```python
from build123d import *

# Parameters (mm, degrees)
SKETCH1_W             = 25.4
SKETCH1_H             = 10.668
BOSS_EXTRUDE1_DEPTH   = 5.334
BOSS_EXTRUDE1_2_DEPTH = 5.334
SKETCH1_3_W           = 329.617035208
SKETCH1_3_H           = 10.668
BOSS_EXTRUDE2_DEPTH   = 12.7
DIHEDRAL_ANGLE_DEPTH  = 5.334
SKETCH3_W             = 50.8
SKETCH3_H             = 12.7
CUT_EXTRUDE1_DEPTH    = 5.334


with BuildPart() as part:
    # Sketch1 → Boss-Extrude1 (new body)
    with BuildSketch(Plane(origin=(0, 5.334, 0), x_dir=(1, 0, 0), z_dir=(0, 1, 0))):
        with Locations((88.9, -59.945526857)):
            Rectangle(SKETCH1_W, SKETCH1_H)
    extrude(amount=-BOSS_EXTRUDE1_DEPTH)



with BuildPart() as body_2:
    # Sketch1 → Boss-Extrude1 2 (new body)
    with BuildSketch(Plane(origin=(0, 5.334, 0), x_dir=(1, 0, 0), z_dir=(0, 1, 0))):
        with Locations((278.817035208, -59.945526857)):
            Rectangle(SKETCH1_W, SKETCH1_H)
    extrude(amount=-BOSS_EXTRUDE1_2_DEPTH)


with BuildPart() as part_1:
    add(part.part)

    add(body_2.part)  # Boss-Extrude2 merges body 2
    # Sketch1<3> → Boss-Extrude2 (add)
    with BuildSketch(Plane(origin=(0, 5.334, 0), x_dir=(1, 0, 0), z_dir=(0, 1, 0))):
        with Locations((164.808517604, -59.945526857)):
            Rectangle(SKETCH1_3_W, SKETCH1_3_H)
    extrude(amount=BOSS_EXTRUDE2_DEPTH)

    # Sketch2 → Dihedral Angle (add)
    with BuildSketch(Plane(origin=(0, 0, 54.611526857), x_dir=(-1, 0, 0), z_dir=(0, 0, -1))):
        Polygon((0, 5.334), (45.946532532, 13.435613355), (43.774704621, 25.752661497), (0, 18.034), align=None)
    extrude(amount=-DIHEDRAL_ANGLE_DEPTH)

    # Sketch3 → Cut-Extrude1 (cut)
    with BuildSketch(Plane.XY.offset(65.279526857)):
        with Locations((25.4, 11.684)):
            Rectangle(SKETCH3_W, SKETCH3_H)
    extrude(amount=-CUT_EXTRUDE1_DEPTH, mode=Mode.SUBTRACT)


solid = part_1.part
```
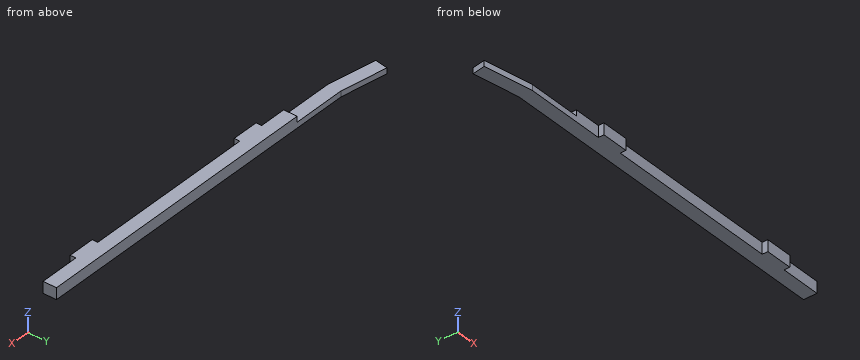
The model under review builds one solid part; all positions refer to its coordinate system, in mm. Give positions to 0.01 mm unless a question says otherwise; leave off trailing zeros. Write each loop counter-clockwise with the first axis right and the second up, starting at its lowest first coordinate (ties: lowest second). Pieces come first, ordered by that corner, then holes. Notation, with made-up numbers: (-15.75, 57.25) - (25.25, 57.25) arc R12 ccw to (25.25, 74.25) - close; hole circle Ø9 at (49, 14.25). An arc over 180 degrees is marked (long way). Answer in a Markdown table with one row per item. Add a question column.
1. We need section D-D on x = 282. Write out the cut boundary in (y, z), then the cut area to 3 significant figures.
2. We need section C-C on y = 10.25. Write out the cut boundary in (x, z), then the cut area to 3 significant figures.
3. Insertion check: P1, Ø2.5, axis at y = 2.5, z = 58, coming from the +X side; P2, Ø2.5, axis at y = 3.5, z = 61, coming from the -X side; P3, Ø3, axis at x = 212.5, z = 58, coming from the -Y side. Each pin has a flat end and moves straight along its axis. Give the tip position at first contact, or say it passes through.
4. We need section A-A on z = 63.5. Write out the cut boundary in (x, y), then the cut area to 3 significant figures.
5. Wall thickness on line 1 along X through (y, z) = (3, 55.5); line 2 along X through (y, z) = (13.25, 64); line 3 along Y through (x, z) = (125, 60): over which ranges is each line inside the solid? List them lowest first. Write a range as [from, to].
6. We need section B-B on x = 16.5. Write out the cut boundary in (y, z), then the cut area to 3 significant figures.
Ans:
| question | item | result |
|---|---|---|
| 1 | outline | (0, 54.61) - (18.03, 54.61) - (18.03, 65.28) - (0, 65.28) - close |
| 1 | area | 192 mm^2 |
| 2 | outline | (-27.88, 54.61) - (329.62, 54.61) - (329.62, 65.28) - (50.8, 65.28) - (50.8, 59.95) - (-27.88, 59.95) - close |
| 2 | area | 3,390 mm^2 |
| 3 | P1 | stops at x = 291.52 |
| 3 | P2 | stops at x = 76.2 |
| 3 | P3 | stops at y = 5.33 |
| 4 | outline | (50.8, 5.33) - (76.2, 5.33) - (76.2, 0) - (101.6, 0) - (101.6, 5.33) - (266.12, 5.33) - (266.12, 0) - (291.52, 0) - (291.52, 5.33) - (329.62, 5.33) - (329.62, 18.03) - (50.8, 18.03) - close |
| 4 | area | 3,810 mm^2 |
| 5 | line 1 | x = [76.2, 101.6], [266.12, 291.52] |
| 5 | line 2 | x = [50.8, 329.62] |
| 5 | line 3 | y = [5.33, 18.03] |
| 6 | outline | (5.33, 54.61) - (18.03, 54.61) - (18.03, 59.95) - (5.33, 59.95) - close |
| 6 | area | 67.7 mm^2 |
